Build history of the part. All positions in model axes, mm. Give positions to 0.01 mm unless a question says otherwise; leave off trailing zeros. Write each loop counter-clockwise with the first axis right and the second up, starting at its lowest first coordinate (ties: lowest second). Pieces come first, ordered by that corner, then holes.
from build123d import *

# Parameters (mm, degrees)
BOSS_EXTRUDE1_DEPTH        = 3.175
F_1_8_0_1250_DOWEL_HOLE1_D = 3.175
SKETCH4_R                  = 4.7625
CUT_EXTRUDE1_DEPTH         = 4.175
M4_CLEARANCE_HOLE1_D       = 4.5
SKETCH7_R                  = 1.5875
CUT_EXTRUDE2_DEPTH         = 4.175
FILLET1_R                  = 4


with BuildPart() as part:
    # Sketch1 → Boss-Extrude1 (new body)
    with BuildSketch(Plane(origin=(0, 0, 0), x_dir=(1, 0, 0), z_dir=(0, 1, 0))):
        with BuildLine():
            Line((4.957224307, 22.517830961), (6.192571563, 13.134436958))
            ThreePointArc((6.192571563, 13.134436958), (8.485281374, 8.485281374), (13.134436958, 6.192571563))
            Line((13.134436958, 6.192571563), (22.517830961, 4.957224307))
            ThreePointArc((22.517830961, 4.957224307), (26.8652, 0), (22.517830961, -4.957224307))
            Line((22.517830961, -4.957224307), (13.134436958, -6.192571563))
            ThreePointArc((13.134436958, -6.192571563), (10.620595205, -6.955137122), (8.485281374, -8.485281374))
            Line((8.485281374, -8.485281374), (-8.485281374, 8.485281374))
            ThreePointArc((-8.485281374, 8.485281374), (-6.955137122, 10.620595205), (-6.192571563, 13.134436958))
            Line((-6.192571563, 13.134436958), (-4.957224307, 22.517830961))
            ThreePointArc((-4.957224307, 22.517830961), (0, 26.8652), (4.957224307, 22.517830961))
        make_face()
    boss_extrude1 = extrude(amount=BOSS_EXTRUDE1_DEPTH)

    # Mirror7: Boss-Extrude1 across plane
    add(boss_extrude1.mirror(Plane(origin=(-8.485281374, 3.175, -8.485281374), x_dir=(0.707106781, 0, 0.707106781), z_dir=(0.707106781, 0, -0.707106781))))

    # 1/8 (0.1250) Dowel Hole1 (through all)
    with Locations(Plane(origin=(0, 3.175, 0), x_dir=(1, 0, 0), z_dir=(0, 1, 0))):
        with Locations((0, 21.8652), (0, -21.8652), (-21.8652, 0), (21.8652, 0)):
            Hole(F_1_8_0_1250_DOWEL_HOLE1_D / 2)

    # Sketch4 → Cut-Extrude1 (cut, through all)
    with BuildSketch(Plane(origin=(0, 3.175, 0), x_dir=(1, 0, 0), z_dir=(0, 1, 0))):
        Circle(SKETCH4_R)
    extrude(amount=-CUT_EXTRUDE1_DEPTH, mode=Mode.SUBTRACT)

    # M4 Clearance Hole1 (through all)
    with Locations(Plane(origin=(0, 3.175, 0), x_dir=(1, 0, 0), z_dir=(0, 1, 0))):
        with Locations((-11.313708499, 0), (0, 11.313708499), (11.313708499, 0), (0, -11.313708499)):
            Hole(M4_CLEARANCE_HOLE1_D / 2)

    # Sketch7 → Cut-Extrude2 (cut, through all)
    with BuildSketch(Plane(origin=(0, 3.175, 0), x_dir=(1, 0, 0), z_dir=(0, 1, 0))):
        with BuildLine():
            ThreePointArc((4.957224307, 22.517830961), (0, 26.8652), (-4.957224307, 22.517830961))
            Line((-4.957224307, 22.517830961), (-5.898887631, 15.365187896))
            ThreePointArc((-5.898887631, 15.365187896), (0, 16.458610949), (5.898887631, 15.365187896))
            Line((5.898887631, 15.365187896), (4.957224307, 22.517830961))
        make_face()
        with Locations((0, 21.8652)):
            Circle(SKETCH7_R, mode=Mode.SUBTRACT)
        with BuildLine():
            ThreePointArc((5.898887631, -15.365187896), (0, -16.458610949), (-5.898887631, -15.365187896))
            Line((-5.898887631, -15.365187896), (-4.957224307, -22.517830961))
            ThreePointArc((-4.957224307, -22.517830961), (0, -26.8652), (4.957224307, -22.517830961))
            Line((4.957224307, -22.517830961), (5.898887631, -15.365187896))
        make_face()
        with Locations((0, -21.8652)):
            Circle(SKETCH7_R, mode=Mode.SUBTRACT)
    extrude(amount=-CUT_EXTRUDE2_DEPTH, mode=Mode.SUBTRACT)

    # Fillet1
    fillet1_edges = [part.edges().sort_by_distance(p)[0] for p in [
        (5.898887631, 1.5875, -15.365187896),
        (-5.898887631, 1.5875, -15.365187896),
        (-5.898887631, 1.5875, 15.365187896),
        (5.898887631, 1.5875, 15.365187896),
    ]]
    fillet(fillet1_edges, radius=FILLET1_R)


solid = part.part
1. Saw through at B-B on z = 0. Give the cut face in (x, y) (1 decimal), plus the area to 3 significant figures.
2. Saw through at C-C on x = -22. Give the cut face in (y, z) (3 decimals), plus the area to 3 significant figures.
3. Drop flat-ended pins along their axis: pin 1 (1 mm diameter, centred on x = 15.5, y = 0.5, fed in from +Z); pin 2 (1.5 mm diameter, centred on y = 2.5, z = 7.5, fed in from -X). Give the stop position or say it passes through.
4. Saw through at D-D on z = -4. Give the cut face in (x, y) (3 decimals), plus the area to 3 significant figures.
5. Saw through at A-A on x = 0. Give the cut face in (y, z) (1 decimal).
6. Drill centre lines: line 1 along X through (y, z) = (0.25, -1); line 2 along Z through (x, y) = (-0.5, 2.6); line 3 along X through (y, z) = (2.7, 2). Where is each one in solid material? Low to high.
7. Mould opens along Z. For faces 1 (the face through (-26.864, 1.565, -0.101)), 2 (the face through (17.892, 1.565, 5.566)), 3 (the face through (23.45, 1.57, -0.07)) say: pulls with the +Z half, pulls with the -Z half, needs draft (parallel to the pull), parting line crosses it, or undercut.
Outcome:
1. outline: (-26.9, 0) - (-23.5, 0) - (-23.5, 3.2) - (-26.9, 3.2) - close; (-20.3, 0) - (-13.6, 0) - (-13.6, 3.2) - (-20.3, 3.2) - close; (-9.1, 0) - (-4.8, 0) - (-4.8, 3.2) - (-9.1, 3.2) - close; (4.8, 0) - (9.1, 0) - (9.1, 3.2) - (4.8, 3.2) - close; (13.6, 0) - (20.3, 0) - (20.3, 3.2) - (13.6, 3.2) - close; (23.5, 0) - (26.9, 0) - (26.9, 3.2) - (23.5, 3.2) - close
1. area: 91.6 mm2
2. outline: (0, -5.025) - (3.175, -5.025) - (3.175, -1.582) - (0, -1.582) - close; (0, 1.582) - (3.175, 1.582) - (3.175, 5.025) - (0, 5.025) - close
2. area: 21.9 mm2
3. pin 1: stops at z = 5.95
3. pin 2: stops at x = -11.07
4. outline: (-24.865, 0) - (-2.585, 0) - (-2.585, 3.175) - (-24.865, 3.175) - close; (2.585, 0) - (24.865, 0) - (24.865, 3.175) - (2.585, 3.175) - close
4. area: 141 mm2
5. outline: (0, -16.5) - (3.2, -16.5) - (3.2, -13.6) - (0, -13.6) - close; (0, -9.1) - (3.2, -9.1) - (3.2, -4.8) - (0, -4.8) - close; (0, 4.8) - (3.2, 4.8) - (3.2, 9.1) - (0, 9.1) - close; (0, 13.6) - (3.2, 13.6) - (3.2, 16.5) - (0, 16.5) - close
6. line 1: x = -26.76 to -23.1, -20.63 to -13.33, -9.3 to -4.66, 4.66 to 9.3, 13.33 to 20.63, 23.1 to 26.76
6. line 2: z = -16.45 to -13.51, -9.12 to -4.74, 4.74 to 9.12, 13.51 to 16.45
6. line 3: x = -26.45 to -12.34, -10.28 to -4.32, 4.32 to 10.28, 12.34 to 26.45
7. face 1: parting line crosses it
7. face 2: pulls with the +Z half
7. face 3: undercut
